Print and shaded views of the part. All mm, measured from the part's lowest x, y and z. Give positions to 0.01 mm unless a question says otherwise; leave off trailing zeros. Write each loop counter-clockwise with the first axis right and the second up, starting at its lowest first coordinate (ties: lowest second). Pieces come first, ordered by that corner, then holes. Notation, with made-up numbers: (88, -25) -> (102, -25) arc R16 ccw to (102, -13) -> close; hole circle Ø8 at (-29.5, 14.25). An arc over 180 degrees is marked (long way). Put each result on its own line as item: value.
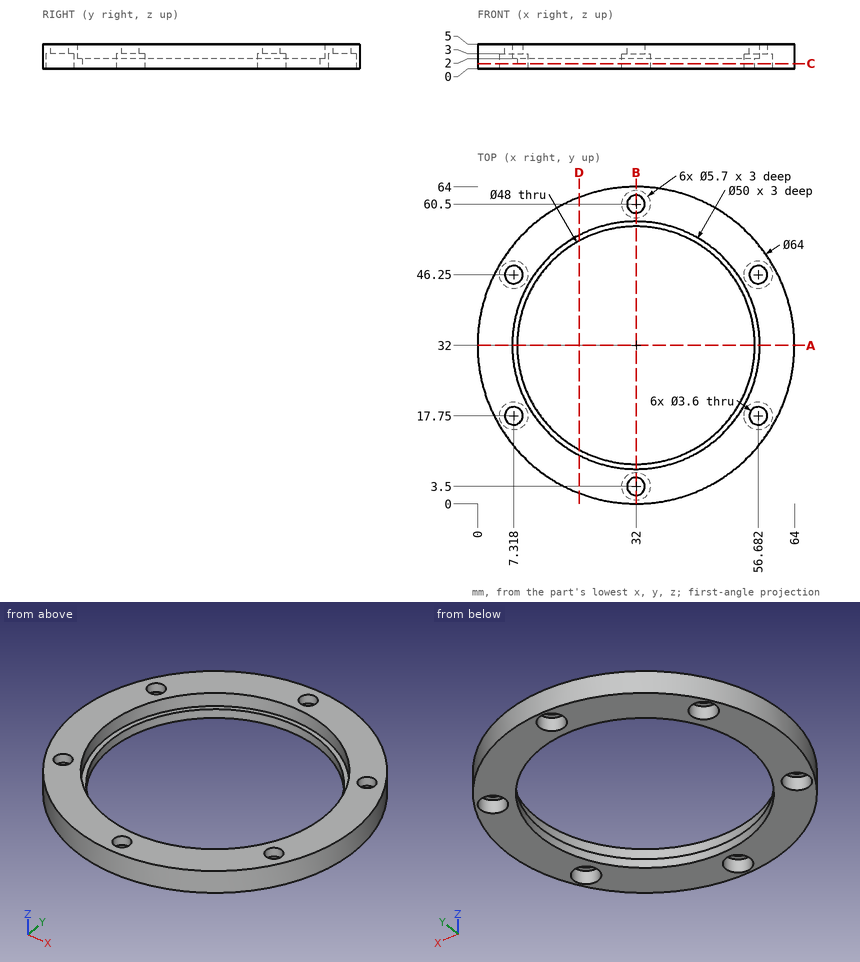
1) Wall check: L1, parallel to Y at x = 32, z = 1.45; L2, parallel to Y at x = 32, z = 4.65; L3, parallel to X at y = 47.5, z = 2.65 (1 decimal). Give the ranges that are in metal, low to high.
Filled sheet:
L1: 0 to 0.65, 6.35 to 8, 56 to 57.65, 63.35 to 64
L2: 0 to 1.7, 5.3 to 7, 57 to 58.7, 62.3 to 64
L3: 4 to 4.8, 9.9 to 12.4, 51.6 to 54.1, 59.2 to 60
2) Slice it at B-B (x = 32). Write the cut outline in (y, z), plus the area to 3 significant figures.
Filled sheet:
outline: (0, 0) -> (0.65, 0) -> (0.65, 3) -> (1.7, 3) -> (1.7, 5) -> (0, 5) -> close; (5.3, 3) -> (6.35, 3) -> (6.35, 0) -> (8, 0) -> (8, 2) -> (7, 2) -> (7, 5) -> (5.3, 5) -> close; (56, 0) -> (57.65, 0) -> (57.65, 3) -> (58.7, 3) -> (58.7, 5) -> (57, 5) -> (57, 2) -> (56, 2) -> close; (62.3, 3) -> (63.35, 3) -> (63.35, 0) -> (64, 0) -> (64, 5) -> (62.3, 5) -> close
area: 25.4 mm2
3) Slice it at D-D (x = 20.5). Write the cut outline in (y, z) (1 decimal).
Filled sheet:
outline: (2.1, 0) -> (10.9, 0) -> (10.9, 2) -> (9.8, 2) -> (9.8, 5) -> (2.1, 5) -> close; (53.1, 0) -> (61.9, 0) -> (61.9, 5) -> (54.2, 5) -> (54.2, 2) -> (53.1, 2) -> close
4) Pin check, flat tips, straight feed: pin 1 (5 mm diameter, centred on x = 56.68, y = 46.25, fed in from -Z); pin 2 (4 mm diameter, centred on x = 56.68, y = 17.75, fed in from +Z); pin 3 (3 mm diameter, centred on x = 52.5, z = 4.5, fed in from +Y); pin 4 (1.5 mm diameter, centred on y = 35, z = 1.5, fed in from -X). Stop position of each tip, or through.
Filled sheet:
pin 1: z = 3
pin 2: z = 5
pin 3: y = 57.75
pin 4: x = 0.08
5) Slice it at C-C (z = 1.05). Write the cut outline in (x, y), plus the area to 3 significant figures.
Filled sheet:
outline: circle Ø64 at (32, 32); hole circle Ø5.7 at (7.32, 17.75); hole circle Ø5.7 at (7.32, 46.25); hole circle Ø48 at (32, 32); hole circle Ø5.7 at (32, 3.5); hole circle Ø5.7 at (32, 60.5); hole circle Ø5.7 at (56.68, 17.75); hole circle Ø5.7 at (56.68, 46.25)
area: 1,250 mm2
6) Slice it at A-A (y = 32). Write the cut outline in (x, z), plus the area to 3 significant figures.
Filled sheet:
outline: (0, 0) -> (8, 0) -> (8, 2) -> (7, 2) -> (7, 5) -> (0, 5) -> close; (56, 0) -> (64, 0) -> (64, 5) -> (57, 5) -> (57, 2) -> (56, 2) -> close
area: 74.0 mm2
